Model file for the job. Use its own axes, mm. A direction names the side the tool comes from. Give positions to 0.01 mm unless a question says otherwise; leave off trailing zeros. Loops run counter-clockwise (first coordinate to the right, second up) from the corner with the lowest first, then second, coordinate; pieces in that order, holes last. Notation, with made-up numbers: M -19.75,67.5 L -0.75,67.5 A6 ccw -0.75,77.5 Z; hole C 9,-36.75 d8. An arc over 180 degrees is marked long. Use CSV: the item, a comma, the result in double quotes. Start each with the question number.
(1) Slice it at C-C on x = -51.5. List the corners of the cut face in (y, z).
(2) Slice it at B-B on x = -21.5. List the corners of the cut face in (y, z).
(3) Two-plate mould, pull along X, no slides. Class faces 1 (the face through (-47, 0, 0)), 2 (the face through (-51.68, 0.49, -21.57)), 3 (the face through (23.85, 0.49, 58.04)): pulls with the +X half, pulls with the -X half, needs draft (parallel to the pull), parting line crosses it, or undercut.
(4) Tool access for faces 4 (the face through (58.04, 0.49, -23.85)), 5 (the face through (39.488, 0.493, 39.708)): list every direction of +Z, -Z, +X, -X, +Y, -Y with a clear straight run to the whole face (end or side of a thin tool).
(5) Flat gauge pin, fed straight in: P1, Ø0.5, axis at x = 49, y = 0.5, coming from the +Z side. Where does the tip first touch, or does it go through?
(6) Wall check: line 1 along Z through (x, y) = (-1, 0.2); line 2 along Z through (x, y) = (48.5, 0.15); line 3 along Z through (x, y) = (-47.5, 0.7). Give the ranges that are in metal, low to high. Write a range as from..to.
(7) Slice it at A-A on z = -7.5. List the corners of the cut face in (x, y), and give its area (3 significant figures).
```python
from build123d import *

# Parameters (mm, degrees)
BOSS_EXTRUDE1_DEPTH = 1
SKETCH2_W           = 10
SKETCH2_H           = 10
BOSS_EXTRUDE2_DEPTH = 1


with BuildPart() as part:
    # Sketch1 → Boss-Extrude1 (new body)
    with BuildSketch(Plane(origin=(0, 0, 0), x_dir=(1, 0, 0), z_dir=(0, 1, 0))):
        Polygon((62.75, -12.481751053), (62.75, 12.481751053), (53.19688133, 35.545019709), (35.545019709, 53.19688133), (12.481751053, 62.75), (-12.481751053, 62.75), (-35.545019709, 53.19688133), (-53.19688133, 35.545019709), (-62.75, 12.481751053), (-62.75, -12.481751053), (-53.19688133, -35.545019709), (-35.545019709, -53.19688133), (-12.481751053, -62.75), (12.481751053, -62.75), (35.545019709, -53.19688133), (53.19688133, -35.545019709), align=None)
        Polygon((56, -11.139092573), (56, 11.139092573), (47.474507641, 31.721451852), (31.721451852, 47.474507641), (11.139092573, 56), (-11.139092573, 56), (-31.721451852, 47.474507641), (-47.474507641, 31.721451852), (-56, 11.139092573), (-56, -11.139092573), (-47.474507641, -31.721451852), (-31.721451852, -47.474507641), (-11.139092573, -56), (11.139092573, -56), (31.721451852, -47.474507641), (47.474507641, -31.721451852), align=None, mode=Mode.SUBTRACT)
    extrude(amount=BOSS_EXTRUDE1_DEPTH)

    # Sketch2 → Boss-Extrude2 (add)
    with BuildSketch(Plane(origin=(0, 1, 0), x_dir=(1, 0, 0), z_dir=(0, 1, 0))):
        with Locations((0, -51)):
            Rectangle(SKETCH2_W, SKETCH2_H)
        with Locations((-51, 0)):
            Rectangle(SKETCH2_W, SKETCH2_H)
        with Locations((0, 51)):
            Rectangle(SKETCH2_W, SKETCH2_H)
        with Locations((51, 0)):
            Rectangle(SKETCH2_W, SKETCH2_H)
    extrude(amount=-BOSS_EXTRUDE2_DEPTH)


solid = part.part
```
Reply:
1,outline,"M 0,-37.24 L 1,-37.24 L 1,-22 L 0,-22 Z; M 0,-5 L 1,-5 L 1,5 L 0,5 Z; M 0,22 L 1,22 L 1,37.24 L 0,37.24 Z"
2,outline,"M 0,-59.01 L 1,-59.01 L 1,-51.71 L 0,-51.71 Z; M 0,51.71 L 1,51.71 L 1,59.01 L 0,59.01 Z"
3,face 1,"needs draft"
3,face 2,"undercut"
3,face 3,"pulls with the +X half"
4,face 4,"-Z, +X, +Y, -Y"
4,face 5,"+Y, -Y"
5,P1,"stops at z = 39.99"
6,line 1,"z = -62.75..-46, 46..62.75"
6,line 2,"z = -40.24..-29.25, -5..5, 29.25..40.24"
6,line 3,"z = -41.24..-31.66, -5..5, 31.66..41.24"
7,outline,"M -62.75,0 L -56,0 L -56,1 L -62.75,1 Z; M 56,0 L 62.75,0 L 62.75,1 L 56,1 Z"
7,area,"13.5 mm^2"
